Autodesk Inventor part; units mm, degrees
ref_plane "Work Plane1" through (8, 0, 0) normal (0, -0.5, -0.866) x (1, 0, 0)
ref_plane "YZ Plane" through (0, 0, 0) normal (1, 0, 0) x (0, 1, 0)
ref_plane "XZ Plane" through (0, 0, 0) normal (0, 1, 0) x (-1, 0, 0)
sketch "Sketch1" plane through (0, 0, 0) normal (0, 0, 1) x (1, 0, 0)
  line L0 (0.5129, 0) -> (12.1667, 0)
  line L1 (16, 1.4434) -> (16, 2.5)
  line L2 (16, 2.5) -> (0, 2.5)
  line L3 (16, 1.4434) -> (13, 1.4434)
  line L4 (13, 1.4434) -> (12.1667, 0)
  line L5 (0, 1.1) -> (0.5129, 0)
  line L6 (0, -0.5) -> (0, 3)
  line L7 (0, 1.1) -> (0, 2.5)
  point P0 (0, 0)
  dimension "d0" = 3
  dimension "d1" = 60
  dimension "d2" = 5
  dimension "d3" = 2.8868
  dimension "d4" = 16
  dimension "d5" = 65
  dimension "d7" = 2.2
revolve "Body" add sketch "Sketch1" angle 360 about axis through (0.5129, 0, 0) along (1, 0, 0)
sketch "Sketch2" plane through (16, 0, 0) normal (1, 0, 0) x (0, 0, -1)
  circle A0 centre (0, 0) radius 1.4434
  circle A1 centre (0, 0) radius 2.5
  line L0 (1.4434, 0) -> (0.7217, -1.25)
  line L1 (0.7217, -1.25) -> (-0.7217, -1.25)
  line L2 (-0.7217, -1.25) -> (-1.4434, 0)
  line L3 (-1.4434, 0) -> (-0.7217, 1.25)
  line L4 (-0.7217, 1.25) -> (0.7217, 1.25)
  line L5 (0.7217, 1.25) -> (1.4434, 0)
extrude "Slot" add sketch "Sketch2" against normal blind 3 contours L5 A0 | A0 L0 | L4 A0 | A0 L1 | L3 A0 | A0 L2
chamfer "Chamfer1" distance 1.4 angle 45 1 edges at (0, -2.5, 0) measured on face at (0, 2.0091, -0.1994)
thread "Thread"
chamfer "Chamfer2" distance 0.4908 angle 45 1 edges at (16, -2.5, 0) measured on face at (11.1332, 2.4919, -0.2012)
ref_plane "Work Plane1" through (8, 0, 0) normal (0, -0.5, -0.866) x (1, 0, 0)
equation "\"d0\" = INTI"
equation "\"d2\" = NND"
equation "\"d3\" = 1.1547 * SW"
equation "\"d4\" = NLG"
equation "\"d5\" = 0.5 * ANG"
equation "\"d7\" = SPD"
equation "\"d8\" = INTI"
equation "\"d10\" = -0.5 * SPD + 0.5 * NND"
equation "\"d11\" = FAWI"
equation "\"d33\" = -0.5 * SPD + 0.5 * NND"
equation "\"d14\" = NLG"
equation "\"d12\" = -0.5 * GD1 + 0.5 * NND"
equation "\"d13\" = FAWI"
equation "\"d34\" = -0.5 * GD1 + 0.5 * NND"
equation "\"NND\" = 5"
equation "\"NLG\" = 16"
equation "\"INTI\" = 3"
equation "\"FAWI\" = 45deg"
equation "\"SW\" = 2.5"
equation "\"GD1\" = THREADDIA - 1.2269 * PTC"
equation "\"ANG\" = 130deg"
equation "\"FAWI1\" = 60deg"
equation "\"SPD\" = 2.2"
equation "\"GUL\" = 0.61345 * PTC"
equation "\"TOA\" = 30deg"
equation "\"THREADDIA\" = 5"
equation "\"PTC\" = 0.8"
equation "\"GAL\" = 0.61345 * PTC"
equation "\"E0\" = 1.155 * SW"
properties part number "AS 1421 - M5 x 16 Cup Point" material "Steel, Mild"
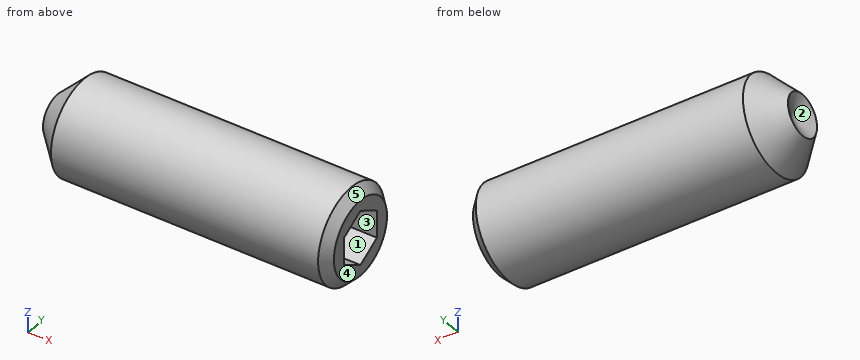
The model under review builds one solid part; all positions refer to its coordinate system, in mm. Face numbers are marked on the shaded views. A direction names the side the tool comes from. Give positions to 0.01 mm unless a question says otherwise; leave off trailing zeros. Order: outer loops, then holes, each group sorted by start corner. A loop starts at its lowest first (then second) coordinate and runs counter-clockwise, first axis right, second up. Notation, with made-up numbers: (88.25, 89) - (106.25, 89) arc R17 cw to (106.25, 96) - close; hole circle Ø3 at (49.5, 75.5). An arc over 180 degrees is marked (long way). Use CSV: the item, a comma, the result in double quotes. Start each with the question number.
Q1. Clearance check with a flat-ended pin moving along its axis: pin 1 Ø1.5 at (x, z) = (8, 2) entering from +Y. State where the tip first meets the part, or that it passes through.
Q2. To check wall thickness, follow line 1 along Z through (x, y) = (13.5, 1.2); line 2 along Z through (x, y) = (13.75, -0.7); line 3 along X through (y, z) = (-0.05, 0.8). State the ranges of each line that lie inside material, in increasing order. Write a range as [from, to].
Q3. The part is to be moulded in two halves that separate along Z. For the marked faces 3, 4 and 5, say which applies: +Z half, -Z half, draft (parallel to the pull), parting line (faces both ways), or undercut.
Q4. Tool access review of the marked faces 1 and 2: name each direction out of +Z, -Z, +X, -X, +Y, -Y from which nothing blocks a thin tool from reaching the whole face with its end or side.
Q5. We need section B-B, the plane x = 6.25. Write out the cut boundary in (y, z).
Q6. We need section A-A, the plane x = 15.25. Write out the cut boundary in (y, z), and give its area (3 significant figures).
Q7. We need section C-C, the plane x = 12.75. Write out the cut boundary in (y, z).
Outcome:
1,pin 1,"stops at y = 2.17"
2,line 1,"z = [-2.19, -0.75], [0.75, 2.19]"
2,line 2,"z = [-2.4, -1.04], [1.04, 2.4]"
2,line 3,"x = [0.14, 12.63]"
3,face 3,"undercut"
3,face 4,"draft"
3,face 5,"parting line"
4,face 1,"+X"
4,face 2,"-X"
5,outline,"circle Ø5 at (0, 0)"
6,outline,"circle Ø5 at (0, 0); hole (-1.25, -0.72) - (0, -1.44) - (1.25, -0.72) - (1.25, 0.72) - (0, 1.44) - (-1.25, 0.72) - close"
6,area,"14.2 mm^2"
7,outline,"circle Ø5 at (0, 0); hole circle Ø2.02 at (0, 0)"
